Geometry: see drawing. Coordinates: mm, zero at the bounding-box minimum. A direction names the side the tool comes from. Round coordinates to 2 decimals unless told otherwise and drop trailing zeros. Write each loop counter-clockwise with the first axis right and the second up, starting at its lowest first coordinate (ties: lowest second). Pieces come first, ordered by that corner, then holes.
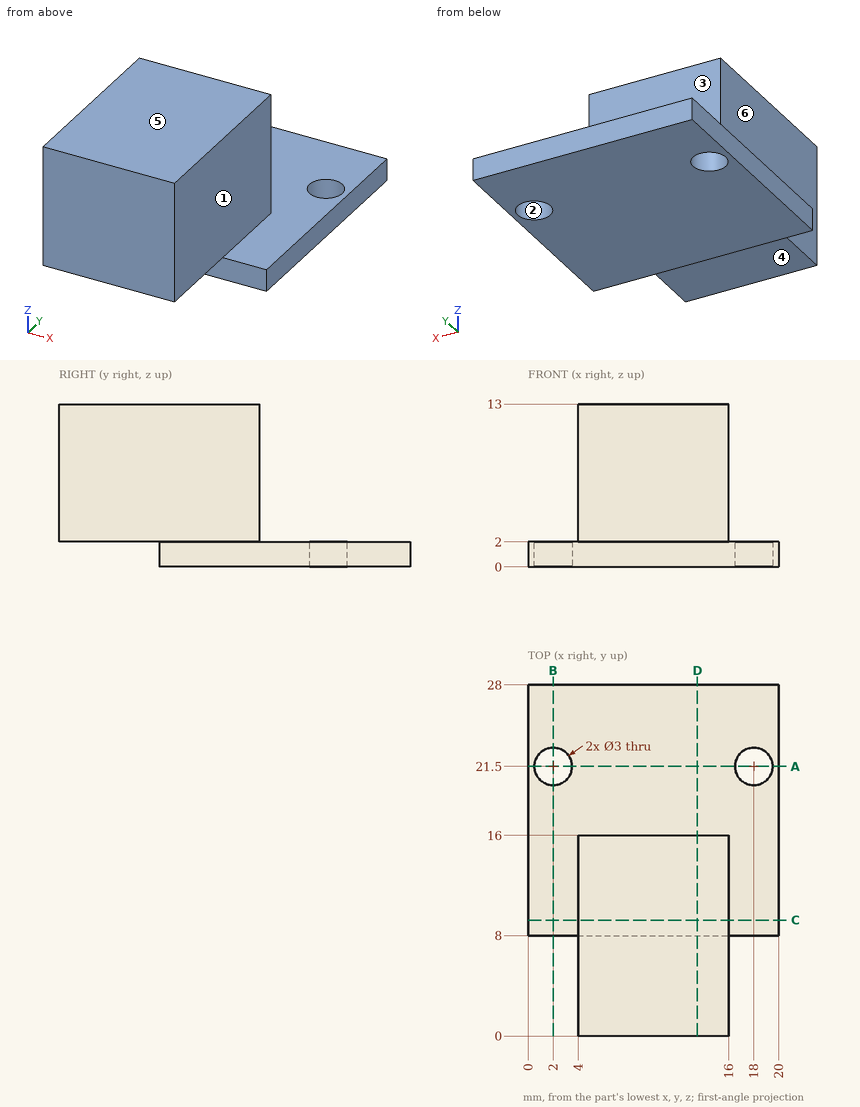
Q1. Line query: line 1 (X direction, y = 21.5, z = 1.25); line 2 (Y direction, x = 2, z = 1); line 3 (Z direction, x = 7.75, y = 21.5). Output: solid intervals per line, ascending.
Q2. Set-up query: the marked faces 4, 5 and 6. Return all of +Z, -Z, +X, -X, +Y, -Y with unobstructed straight access to the full face (end or side cutting, diameter ignored); none if empty.
Q3. Section query A-A, the plane y = 21.5. Output: boundary loops of the cut face in (x, z).
Q4. Mould query, pull axis Y, two halves, no side actions, for the marked faces 1, 2 and 3. Classes: pulls with the +Y half, pulls with the -Y half, needs draft (parallel to the pull), parting line crosses it, or undercut.
Q5. Section query D-D, the plane x = 13.5. Output: boundary loops of the cut face in (y, z).
Q6. Section query C-C, the plane y = 9.25. Output: boundary loops of the cut face in (x, z).
Q7. Pin query (flat end, axial travel): P1, Ø3, axis at y = 12.5, z = 7, coming from the -X side; P2, Ø4, axis at x = 16, z = 6.5, coming from the +Y side; P3, Ø3.5, axis at y = 10, z = 10, coming from the +X side. Return the tip coordinate at first contact, or that it passes through.
Q8. Section query B-B, the plane x = 2. Output: boundary loops of the cut face in (y, z).
Filled in:
1. line 1: x = 0 to 0.5, 3.5 to 16.5, 19.5 to 20
1. line 2: y = 8 to 20, 23 to 28
1. line 3: z = 0 to 2
2. face 4: -Z, +X, -X, -Y
2. face 5: +Z, +X, -X, +Y, -Y
2. face 6: +Z, -X, +Y, -Y
3. outline: (0, 0) - (0.5, 0) - (0.5, 2) - (0, 2) - close; (3.5, 0) - (16.5, 0) - (16.5, 2) - (3.5, 2) - close; (19.5, 0) - (20, 0) - (20, 2) - (19.5, 2) - close
4. face 1: needs draft
4. face 2: undercut
4. face 3: pulls with the +Y half
5. outline: (0, 2) - (8, 2) - (8, 0) - (28, 0) - (28, 2) - (16, 2) - (16, 13) - (0, 13) - close
6. outline: (0, 0) - (20, 0) - (20, 2) - (16, 2) - (16, 13) - (4, 13) - (4, 2) - (0, 2) - close
7. P1: stops at x = 4
7. P2: stops at y = 16
7. P3: stops at x = 16
8. outline: (8, 0) - (20, 0) - (20, 2) - (8, 2) - close; (23, 0) - (28, 0) - (28, 2) - (23, 2) - close
